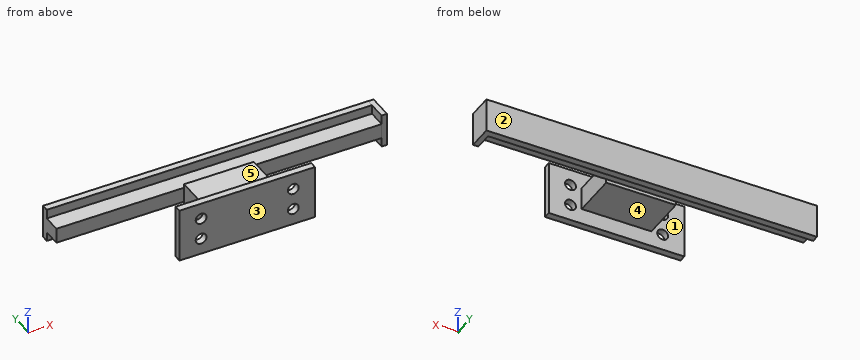
from build123d import *

# Parameters (mm, degrees)
SKETCH1_W           = 50
SKETCH1_H           = 20
SKETCH1_R           = 2
BOSS_EXTRUDE1_DEPTH = 2.54
SKETCH2_W           = 25.697892262
SKETCH2_H           = 8.354695914
BOSS_EXTRUDE2_DEPTH = 16.51
SKETCH3_W           = 120
SKETCH3_H           = 5.588
BOSS_EXTRUDE3_DEPTH = 6.51
SKETCH4_W           = 120
SKETCH4_H           = 12.446
BOSS_EXTRUDE4_DEPTH = 2.54
SKETCH6_W           = 12.425038184
SKETCH6_H           = 9.042273223
BOSS_EXTRUDE6_DEPTH = 2


with BuildPart() as part:
    # Sketch1 → Boss-Extrude1 (new body)
    with BuildSketch(Plane(origin=(0, 0, 0), x_dir=(1, 0, 0), z_dir=(0, 1, 0))):
        with Locations((0, -2.5)):
            Rectangle(SKETCH1_W, SKETCH1_H)
        with Locations(Location((17, -6.5, 0), (0, 0, 270))):
            Circle(SKETCH1_R, mode=Mode.SUBTRACT)
        with Locations(Location((17, 1.5, 0), (0, 0, 270))):
            Circle(SKETCH1_R, mode=Mode.SUBTRACT)
        with Locations(Location((-17, -6.5, 0), (0, 0, 270))):
            Circle(SKETCH1_R, mode=Mode.SUBTRACT)
        with Locations(Location((-17, 1.5, 0), (0, 0, 270))):
            Circle(SKETCH1_R, mode=Mode.SUBTRACT)
    extrude(amount=BOSS_EXTRUDE1_DEPTH)

    # Sketch2 → Boss-Extrude2 (add)
    with BuildSketch(Plane(origin=(0, 2.54, 0), x_dir=(1, 0, 0), z_dir=(0, 1, 0))):
        with Locations((0, -2.5)):
            Rectangle(SKETCH2_W, SKETCH2_H)
    extrude(amount=BOSS_EXTRUDE2_DEPTH)

    # Sketch3 → Boss-Extrude3 (add)
    with BuildSketch(Plane(origin=(0, 19.05, 0), x_dir=(1, 0, 0), z_dir=(0, 1, 0))):
        with Locations((0, -2.5)):
            Rectangle(SKETCH3_W, SKETCH3_H)
    extrude(amount=BOSS_EXTRUDE3_DEPTH)

    # Sketch4 → Boss-Extrude4 (add)
    with BuildSketch(Plane(origin=(0, 25.56, 0), x_dir=(1, 0, 0), z_dir=(0, 1, 0))):
        with Locations((0, -2.5)):
            Rectangle(SKETCH4_W, SKETCH4_H)
    extrude(amount=BOSS_EXTRUDE4_DEPTH)

    # Sketch6 → Boss-Extrude6 (add)
    with BuildSketch(Plane(origin=(60, 0, 0), x_dir=(0, 0, -1), z_dir=(1, 0, 0))):
        with Locations((-2.489519092, 23.578863389)):
            Rectangle(SKETCH6_W, SKETCH6_H)
    extrude(amount=BOSS_EXTRUDE6_DEPTH)


solid = part.part
Verification items for the finished model (mm, model axes). Face numbers are marked on the shaded views. A direction names the side the tool comes from. Coordinates: 2 decimals unless noted, no trailing zeros. Order: outer loops, then holes, each group sorted by start corner. A loop starts at its lowest first (then second) coordinate and runs counter-clockwise, first axis right, second up.
1. Release check for a two-part mould opening along Y. For the marked faces 1, 2 and 3 record: +Y half, -Y half, draft (parallel to the pull), parting line (faces both ways), or undercut.
Results found:
face 1: undercut
face 2: +Y half
face 3: -Y half
2. Sectioned sample at D-D, the plane z = 11. Record the cut outline in (x, y).
Results found:
outline: (-25, 0) - (25, 0) - (25, 2.54) - (-25, 2.54) - close
3. Set-up check for the marked faces 4 and 5: record each of +Z, -Z, +X, -X, +Y, -Y from which the full face is reachable in a straight line by a thin tool's end or side.
Results found:
face 4: -Z, +X, -X
face 5: +Z, +X, -X
4. Go/stop test with flat-tipped pins: pin 1 Ø5 at (x, y) = (3, 8) entering from +Z; pin 2 Ø1.5 at (x, z) = (41.5, -2) entering from -Y; pin 3 Ø6 at (x, z) = (-32, 1.5) entering from -Y; pin 4 Ø10 at (x, y) = (-23, 6.5) entering from +Z. Record where each tip stops, or that it passes through.
Results found:
pin 1: stops at z = 6.68
pin 2: stops at y = 25.56
pin 3: stops at y = 19.05
pin 4: stops at z = 12.5
5. Scan lines: line 1 (X direction, y = 2.05, z = 6.5); line 2 (Z direction, x = 47, y = 22.5); line 3 (Y direction, x = 16.5, z = 1.5). Record each from-to range of solid material in increasing order.
Results found:
line 1: x = -25 to -19, -15 to 15, 19 to 25
line 2: z = -0.29 to 5.29
line 3: y = 0 to 2.54, 19.05 to 28.1
6. Sectioned sample at C-C, the plane x = 38. Record the cut outline in (y, z), and give its area (3 significant figures).
Results found:
outline: (19.05, -0.29) - (25.56, -0.29) - (25.56, -3.72) - (28.1, -3.72) - (28.1, 8.72) - (25.56, 8.72) - (25.56, 5.29) - (19.05, 5.29) - close
area: 68.0 mm2
7. Sectioned sample at B-B, the plane x = -17. Record the cut outline in (y, z), and give its area (3 significant figures).
Results found:
outline: (0, -7.5) - (2.54, -7.5) - (2.54, -3.5) - (0, -3.5) - close; (0, 0.5) - (2.54, 0.5) - (2.54, 4.5) - (0, 4.5) - close; (0, 8.5) - (2.54, 8.5) - (2.54, 12.5) - (0, 12.5) - close; (19.05, -0.29) - (25.56, -0.29) - (25.56, -3.72) - (28.1, -3.72) - (28.1, 8.72) - (25.56, 8.72) - (25.56, 5.29) - (19.05, 5.29) - close
area: 98.5 mm2
8. Sectioned sample at A-A, the plane y = 23.25. Record the cut outline in (x, z).
Results found:
outline: (-60, -0.29) - (60, -0.29) - (60, -3.72) - (62, -3.72) - (62, 8.7) - (60, 8.7) - (60, 5.29) - (-60, 5.29) - close
